Design review of the part shown in the three views and the two pictorial views. Dimensions are in mm from the part's minimum x, y and z. Give positions to 0.01 mm unless a question says otherwise; leave off trailing zeros. Loops run counter-clockwise (first coordinate to the right, second up) from the corner with the lowest first, then second, coordinate; pieces in that order, holes last.
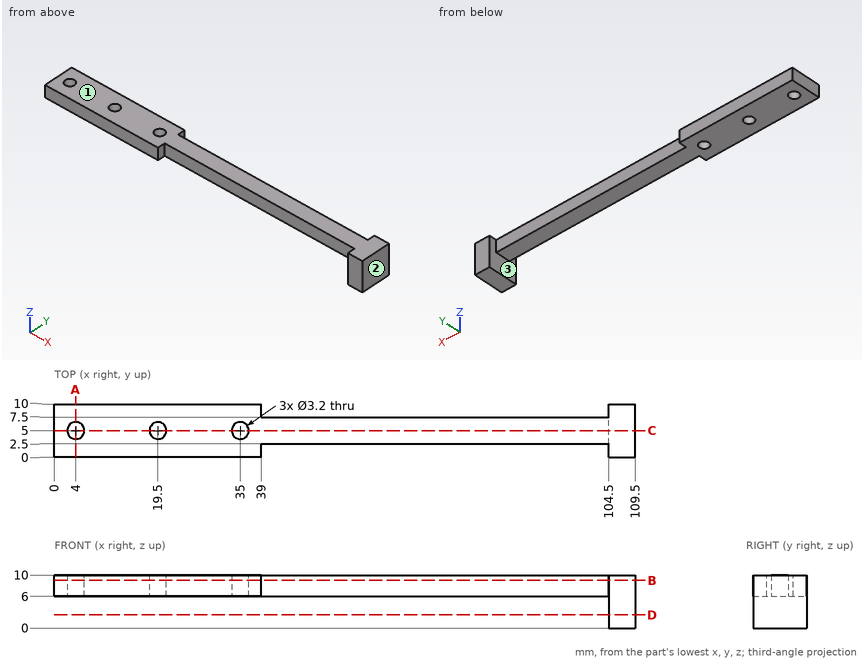
Q1. Draft analysis for pull direction X (two halves, no side actions). For the marked faces 1, 2 and 3, state which applies: pulls with the +X half, pulls with the -X half, needs draft (parallel to the pull), parting line crosses it, or undercut.
Results:
face 1: needs draft
face 2: pulls with the +X half
face 3: undercut
Q2. Take a section at B-B (z = 9). Give the boundary of the cut face in (x, y).
Results:
outline: (0, 0) - (39, 0) - (39, 2.5) - (104.5, 2.5) - (104.5, 0) - (109.5, 0) - (109.5, 10) - (104.5, 10) - (104.5, 7.5) - (39, 7.5) - (39, 10) - (0, 10) - close; hole circle Ø3.2 at (4, 5); hole circle Ø3.2 at (19.5, 5); hole circle Ø3.2 at (35, 5)
Q3. Take a section at D-D (z = 2.5). Give the boundary of the cut face in (x, y), plus the area to 3 significant figures.
Results:
outline: (104.5, 0) - (109.5, 0) - (109.5, 10) - (104.5, 10) - close
area: 50.0 mm2
Q4. Take a section at A-A (x = 4). Give the boundary of the cut face in (y, z), plus the area to 3 significant figures.
Results:
outline: (0, 6) - (3.4, 6) - (3.4, 10) - (0, 10) - close; (6.6, 6) - (10, 6) - (10, 10) - (6.6, 10) - close
area: 27.2 mm2
Q5. Insertion check: pin 1 (4 mm diameter, centred on x = 43, z = 6, fed in from +Y); pin 2 (1.5 mm diameter, centred on x = 63, y = 7.5, fed in from -Z); pin 3 (3 mm diameter, centred on y = 5.5, z = 4, fed in from -X). Each pin has a flat end and moves straight along its axis. Give the tip position at first contact, or say it passes through.
Results:
pin 1: stops at y = 7.5
pin 2: stops at z = 6
pin 3: stops at x = 104.5
Q6. Take a section at C-C (y = 5). Give the boundary of the cut face in (x, z).
Results:
outline: (0, 6) - (2.4, 6) - (2.4, 10) - (0, 10) - close; (5.6, 6) - (17.9, 6) - (17.9, 10) - (5.6, 10) - close; (21.1, 6) - (33.4, 6) - (33.4, 10) - (21.1, 10) - close; (36.6, 6) - (104.5, 6) - (104.5, 0) - (109.5, 0) - (109.5, 10) - (36.6, 10) - close
Q7. Wall thickness on line 1 (Y direction, x = 4, z = 7.9); line 2 (X direction, y = 5.5, z = 9.75); line 3 (Z direction, x = 39.5, y = 5.5): over which ranges is each line inside the solid? List them lowest first.
Results:
line 1: y = 0 to 3.4, 6.6 to 10
line 2: x = 0 to 2.48, 5.52 to 17.98, 21.02 to 33.48, 36.52 to 109.5
line 3: z = 6 to 10
